The drawing under review shows one solid part. Ordinate dimensions are in mm from its lowest x, y, z. A direction names the side the tool comes from. Round coordinates to 2 decimals unless told otherwise and drop trailing zeros. Order: outer loops, then holes, each group sorted by start corner. A loop starts at its lowest first (then second) coordinate and runs counter-clockwise, first axis right, second up.
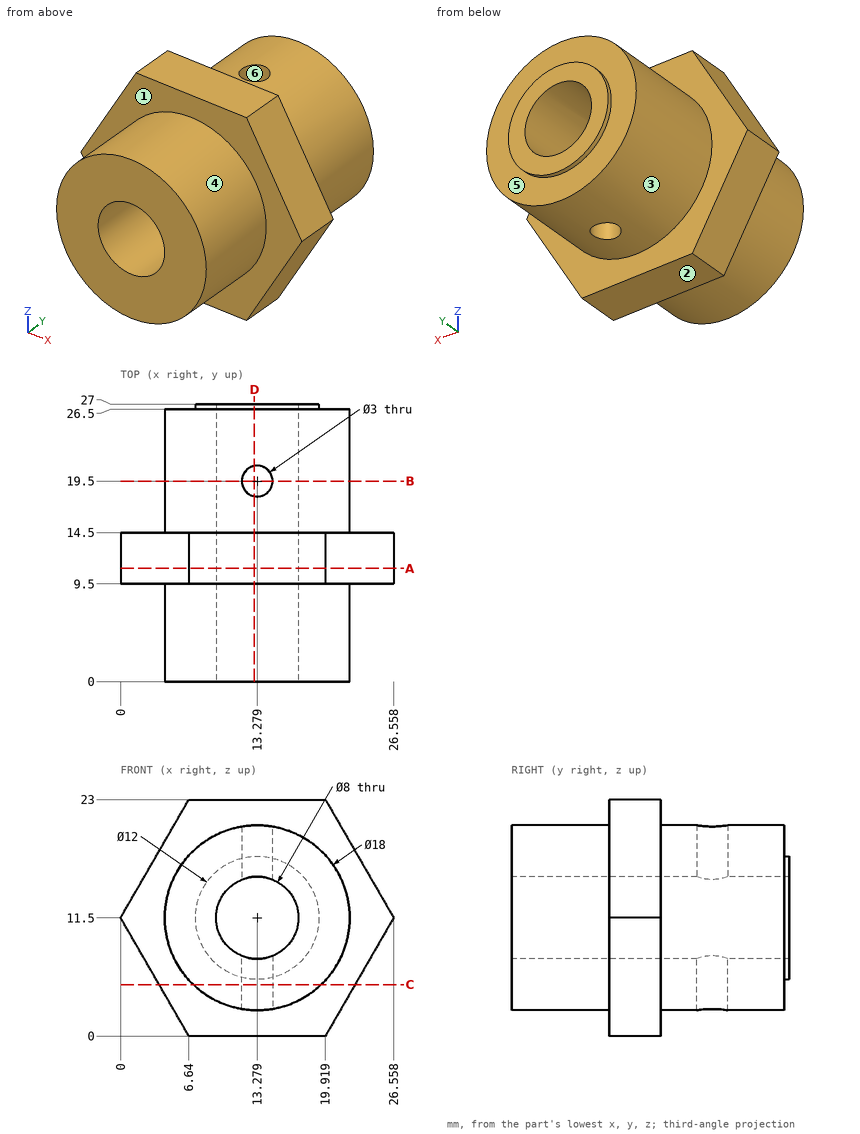
(1) We need section B-B (y = 19.5). Give the boundary of the cut face in (x, z) (1 decimal).
(2) The part is to be moulded in two halves that separate along X. For the marked faces 4, 5 and 6, say which applies: pulls with the +X half, pulls with the -X half, needs draft (parallel to the pull), parting line crosses it, or undercut.
(3) We need section C-C (z = 5). Give the boundary of the cut face in (x, y) (1 decimal), and give its area (3 significant figures).
(4) We need section D-D (x = 13). Give the boundary of the cut face in (y, z) (1 decimal), and give its area (3 significant figures).
(5) We need section A-A (y = 11). Give the boundary of the cut face in (x, z).
(6) Clearance check with flat-ended pins moving along their axes: P1, Ø1.5, axis at y = 20.5, z = 17.5, coming from the -X side; P2, Ø5, axis at y = 3.5, z = 10, coming from the +X side; P3, Ø2, axis at y = 23.5, z = 18, coming from the -X side (1 decimal). State where each tip first meets the part, or that it passes through.
(7) To check wall thickness, follow L1, parallel to X at y = 25.25, z = 11.5; L2, parallel to Z at x = 13.5, y = 25; L3, parallel to X at y = 13.5, z = 11.5. State the ranges of each line that lie inside material, in increasing order.
(8) Tool access review of the marked faces 1, 2 and 3: name each direction out of +Z, -Z, +X, -X, +Y, -Y from which nothing blocks a thin tool from reaching the whole face with its end or side.
Verdict:
1. outline: (11.8, 2.6) - (11.8, 7.8) arc R4 cw to (11.8, 15.2) - (11.8, 20.4) arc R9 ccw to start; (14.8, 2.6) arc R9 ccw to (14.8, 20.4) - (14.8, 15.2) arc R4 cw to (14.8, 7.8) - close
2. face 4: parting line crosses it
2. face 5: needs draft
2. face 6: undercut
3. outline: (3.8, 9.5) - (7.1, 9.5) - (7.1, 0) - (19.5, 0) - (19.5, 9.5) - (22.8, 9.5) - (22.8, 14.5) - (19.5, 14.5) - (19.5, 26.5) - (7.1, 26.5) - (7.1, 14.5) - (3.8, 14.5) - close; hole circle Ø3 at (13.3, 19.5)
3. area: 356 mm2
4. outline: (0, 2.5) - (9.5, 2.5) - (9.5, 0) - (14.5, 0) - (14.5, 2.5) - (18, 2.5) - (18, 7.5) - (0, 7.5) - close; (0, 15.5) - (18, 15.5) - (18, 20.5) - (14.5, 20.5) - (14.5, 23) - (9.5, 23) - (9.5, 20.5) - (0, 20.5) - close; (21, 2.5) - (26.5, 2.5) - (26.5, 5.5) - (27, 5.5) - (27, 7.5) - (21, 7.5) - close; (21, 15.5) - (27, 15.5) - (27, 17.5) - (26.5, 17.5) - (26.5, 20.5) - (21, 20.5) - close
4. area: 263 mm2
5. outline: (0, 11.5) - (6.64, 0) - (19.92, 0) - (26.56, 11.5) - (19.92, 23) - (6.64, 23) - close; hole circle Ø8 at (13.28, 11.5)
6. P1: stops at x = 5.97
6. P2: stops at x = 22.28
6. P3: stops at x = 6.2
7. L1: x = 4.28 to 9.28, 17.28 to 22.28
7. L2: z = 2.5 to 7.51, 15.49 to 20.5
7. L3: x = 0 to 9.28, 17.28 to 26.56
8. face 1: -Y
8. face 2: -Z, +X, -X, +Y, -Y
8. face 3: +Y
